Part model, mm, in its own coordinate system. Give positions to 0.01 mm unless a question says otherwise; leave off trailing zeros. Write each loop counter-clockwise with the first axis right and the second up, starting at its lowest first coordinate (ties: lowest second). Pieces come first, ordered by that corner, then holes.
```python
from build123d import *

# Parameters (mm, degrees)
F0_W     = 87
F0_H     = 42
F0_R     = 1.75
F0_W_2   = 28.5
F0_H_2   = 11
F0_R_2   = 2.5
F1_DEPTH = 2
F2_R     = 3


with BuildPart() as f1:
    # F0 (on Front) → F1 (new body)
    with BuildSketch(Plane.XZ):
        Rectangle(F0_W, F0_H)
        with Locations((-40, -17.5)):
            Circle(F0_R, mode=Mode.SUBTRACT)
        with Locations((-19.25, -10.5)):
            Rectangle(F0_W_2, F0_H_2, mode=Mode.SUBTRACT)
        with Locations((40, -17.5)):
            Circle(F0_R, mode=Mode.SUBTRACT)
        with Locations((19.25, -10.5)):
            Rectangle(F0_W_2, F0_H_2, mode=Mode.SUBTRACT)
        with Locations((-40, 9.5)):
            Circle(F0_R_2, mode=Mode.SUBTRACT)
        with Locations((-40, 17.5)):
            Circle(F0_R, mode=Mode.SUBTRACT)
        with Locations((-19.25, 10.5)):
            Rectangle(F0_W_2, F0_H_2, mode=Mode.SUBTRACT)
        with Locations((40, 9.5)):
            Circle(F0_R_2, mode=Mode.SUBTRACT)
        with Locations((19.25, 10.5)):
            Rectangle(F0_W_2, F0_H_2, mode=Mode.SUBTRACT)
        with Locations((40, 17.5)):
            Circle(F0_R, mode=Mode.SUBTRACT)
    extrude(amount=F1_DEPTH)

    # F2
    f2_edges = [f1.edges().sort_by_distance(p)[0] for p in [
        (-43.5, -1, 21),
        (-43.5, -1, -21),
        (43.5, -1, -21),
        (43.5, -1, 21),
        (-5, -1, 16),
        (33.5, -1, 16),
        (-33.5, -1, 16),
        (-33.5, -1, -5),
        (5, -1, -5),
        (5, -1, 16),
        (-33.5, -1, -16),
        (-33.5, -1, 5),
        (5, -1, 5),
        (5, -1, -16),
        (33.5, -1, 5),
        (33.5, -1, -16),
        (-5, -1, 5),
        (-5, -1, -5),
        (-5, -1, -16),
        (33.5, -1, -5),
    ]]
    fillet(f2_edges, radius=F2_R)


solid = f1.part
```
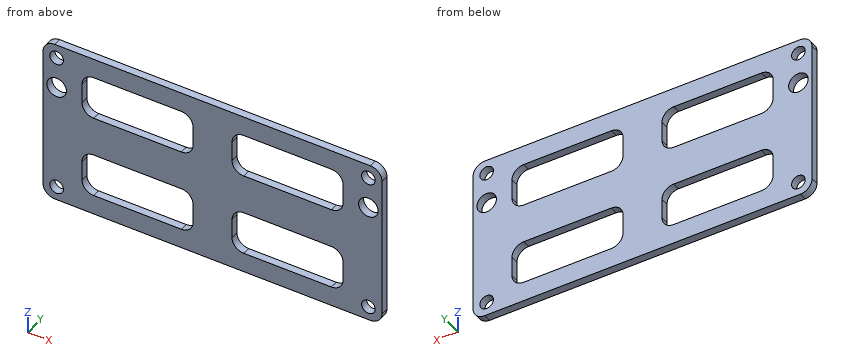
1) Pin check, flat tip, straight feed: pin 1 Ø1.5 at (x, z) = (-10, 15) entering from -Y. Stop position of the tip, or through.
Answers follow:
pin 1: passes through
2) Saw through at B-B, the plane y = -0.7. Count the separate pieces of the cut face and the enclosed holes in it, then the cut area to 3 significant figures.
Answers follow:
separate pieces: 1
enclosed holes: 10
area: 2,350 mm2
3) Wall check: L1, parallel to Z at x = -14.5, y = -1; L2, parallel to Z at x = -40, y = -0.9; L3, parallel to X at y = -1.35, z = -13. Give the ranges that are in metal, low to high.
Answers follow:
L1: z = -21 to -16, -5 to 5, 16 to 21
L2: z = -21 to -19.25, -15.75 to 7, 12 to 15.75, 19.25 to 21
L3: x = -43.5 to -33.5, -5 to 5, 33.5 to 43.5
4) Saw through at A-A, the plane x = -14.5. Write the cut outline in (y, z).
Answers follow:
outline: (-2, -21) - (0, -21) - (0, -16) - (-2, -16) - close; (-2, -5) - (0, -5) - (0, 5) - (-2, 5) - close; (-2, 16) - (0, 16) - (0, 21) - (-2, 21) - close
